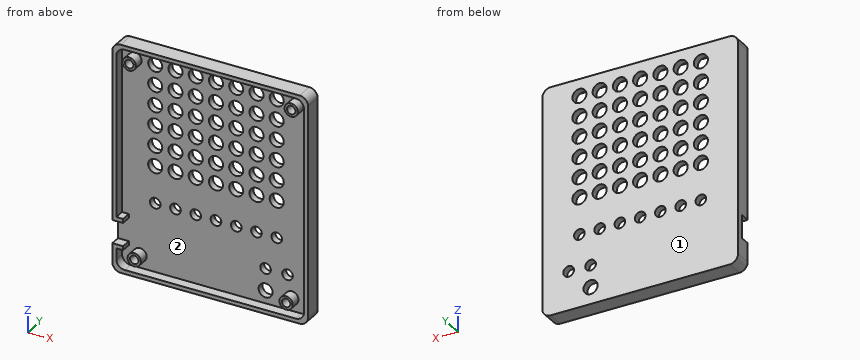
Autodesk Inventor part; units mm, degrees
ref_plane "YZ Plane" through (0, 0, 0) normal (1, 0, 0) x (0, 1, 0)
ref_plane "XZ Plane" through (0, 0, 0) normal (0, 1, 0) x (-1, 0, 0)
ref_plane "XY Plane" through (0, 0, 0) normal (0, 0, 1) x (1, 0, 0)
sketch "Sketch1" plane through (0, 0, 0) normal (0, 1, 0) x (-1, 0, 0)
  line L0 (-2.54, -83.185) -> (-71.12, -83.185) construction
  line L1 (-71.12, -83.185) -> (-71.12, -2.54) construction
  line L2 (-71.12, -2.54) -> (-2.54, -2.54) construction
  line L3 (-2.54, -2.54) -> (-2.54, -83.185) construction
  line L4 (0, -85.725) -> (-73.66, -85.725)
  line L5 (-73.66, -85.725) -> (-73.66, 0)
  line L6 (-73.66, 0) -> (0, 0)
  line L7 (0, 0) -> (0, -85.725)
  line L8 (-2.54, -83.185) -> (0, -85.725) construction
  line L9 (-71.12, -83.185) -> (-73.66, -85.725) construction
  line L10 (-73.66, 0) -> (-71.12, -2.54) construction
  line L11 (-2.54, -2.54) -> (0, 0) construction
  line L12 (-1.5, -84.225) -> (-72.16, -84.225)
  line L13 (-72.16, -84.225) -> (-72.16, -1.5)
  line L14 (-72.16, -1.5) -> (-1.5, -1.5)
  line L15 (-1.5, -1.5) -> (-1.5, -84.225)
  circle A0 centre (-8.255, -79.375) radius 1.6
  circle A1 centre (-65.405, -79.375) radius 1.6
  circle A2 centre (-6.35, -6.35) radius 1.6
  circle A3 centre (-67.31, -6.35) radius 1.6
  line L16 (-8.255, -79.375) -> (-65.405, -79.375) construction
  line L17 (-67.31, -6.35) -> (-6.35, -6.35) construction
  line L18 (-6.35, -6.35) -> (-8.255, -79.375) construction
  line L19 (-65.405, -79.375) -> (-67.31, -6.35) construction
  circle A4 centre (-8.255, -79.375) radius 2.5
  circle A5 centre (-65.405, -79.375) radius 2.5
  circle A6 centre (-67.31, -6.35) radius 2.5
  circle A7 centre (-6.35, -6.35) radius 2.5
  point P0 (0, 0)
  dimension "d0" = 68.58
  dimension "d1" = 80.645
  dimension "d2" = 2.54
  dimension "d3" = 2.54
  dimension "d4" = 1.5
  dimension "d5" = 57.15
  dimension "d6" = 60.96
  dimension "d7" = 73.025
  dimension "d9" = 3.81
  dimension "d10" = 3.81
  dimension "d11" = 3.81
  dimension "d12" = 3.2
  dimension "d13" = 5
extrude "Extrusion1" add sketch "Sketch1" along normal blind 2.54 contours L4 L5 L6 L7 | L12 L13 L14 L15 | A0 | A1 | A2 | A3 | A4 | A5 | A6 | A7
extrude "Extrusion2" add sketch "Sketch1" against normal blind 3.81
sketch "Sketch2" plane through (0, 0, 0) normal (0, -1, 0) x (1, 0, 0)
  circle A0 centre (67.31, -6.35) radius 2.5
  circle A1 centre (8.255, -79.375) radius 2.5
  line L0 (1.5, -1.5) -> (1.5, -84.225)
  line L1 (1.5, -84.225) -> (72.16, -84.225)
  line L2 (72.16, -84.225) -> (72.16, -1.5)
  line L3 (72.16, -1.5) -> (1.5, -1.5)
  circle A2 centre (65.405, -79.375) radius 2.5
  circle A3 centre (6.35, -6.35) radius 2.5
  circle A4 centre (59.69, -6.35) radius 2.65
  circle A5 centre (59.69, -13.97) radius 2.65
  circle A6 centre (59.69, -21.59) radius 2.65
  circle A7 centre (59.69, -29.21) radius 2.65
  circle A8 centre (59.69, -36.83) radius 2.65
  circle A9 centre (59.69, -44.45) radius 2.65
  circle A10 centre (52.07, -6.35) radius 2.65
  circle A11 centre (52.07, -13.97) radius 2.65
  circle A12 centre (52.07, -21.59) radius 2.65
  circle A13 centre (52.07, -29.21) radius 2.65
  circle A14 centre (52.07, -36.83) radius 2.65
  circle A15 centre (52.07, -44.45) radius 2.65
  circle A16 centre (44.45, -6.35) radius 2.65
  circle A17 centre (44.45, -13.97) radius 2.65
  circle A18 centre (44.45, -21.59) radius 2.65
  circle A19 centre (44.45, -29.21) radius 2.65
  circle A20 centre (44.45, -36.83) radius 2.65
  circle A21 centre (44.45, -44.45) radius 2.65
  circle A22 centre (36.83, -6.35) radius 2.65
  circle A23 centre (36.83, -13.97) radius 2.65
  circle A24 centre (36.83, -21.59) radius 2.65
  circle A25 centre (36.83, -29.21) radius 2.65
  circle A26 centre (36.83, -36.83) radius 2.65
  circle A27 centre (36.83, -44.45) radius 2.65
  circle A28 centre (29.21, -6.35) radius 2.65
  circle A29 centre (29.21, -13.97) radius 2.65
  circle A30 centre (29.21, -21.59) radius 2.65
  circle A31 centre (29.21, -29.21) radius 2.65
  circle A32 centre (29.21, -36.83) radius 2.65
  circle A33 centre (29.21, -44.45) radius 2.65
  circle A34 centre (21.59, -6.35) radius 2.65
  circle A35 centre (21.59, -13.97) radius 2.65
  circle A36 centre (21.59, -21.59) radius 2.65
  circle A37 centre (21.59, -29.21) radius 2.65
  circle A38 centre (21.59, -36.83) radius 2.65
  circle A39 centre (21.59, -44.45) radius 2.65
  circle A40 centre (13.97, -6.35) radius 2.65
  circle A41 centre (13.97, -13.97) radius 2.65
  circle A42 centre (13.97, -21.59) radius 2.65
  circle A43 centre (13.97, -29.21) radius 2.65
  circle A44 centre (13.97, -36.83) radius 2.65
  circle A45 centre (13.97, -44.45) radius 2.65
  circle A46 centre (59.69, -58.3946) radius 2
  circle A47 centre (52.07, -58.3946) radius 2
  circle A48 centre (44.45, -58.3946) radius 2
  circle A49 centre (36.83, -58.3946) radius 2
  circle A50 centre (29.21, -58.3946) radius 2
  circle A51 centre (21.59, -58.3946) radius 2
  circle A52 centre (13.97, -58.3946) radius 2
  line L4 (67.31, -6.35) -> (59.69, -6.35) construction
  line L5 (65.405, -79.375) -> (59.69, -58.3946) construction
  line L6 (13.97, -58.3946) -> (8.255, -79.375) construction
  circle A53 centre (55.499, -79.375) radius 2.65
  line L7 (55.499, -79.375) -> (65.405, -79.375) construction
  circle A54 centre (55.499, -71.1454) radius 2
  circle A55 centre (63.754, -71.1454) radius 2
  line L8 (55.499, -71.1454) -> (63.754, -71.1454) construction
  line L9 (55.499, -71.1454) -> (55.499, -79.375) construction
  point P0 (0, 0)
  dimension "d20" = 7.62
  dimension "d23" = 7.62
  dimension "d26" = 5.3
  dimension "d29" = 7.62
  dimension "d34" = 7.62
  dimension "d35" = 7.62
  dimension "d36" = 60.96
  dimension "d37" = 20.9804
  dimension "d38" = 4
  dimension "d40" = 9.906
  dimension "d41" = 8.255
  dimension "d42" = 8.2296
extrude "Extrusion3" cut sketch "Sketch2" against normal through all contours A4 | A5 | A6 | A7 | A8 | A9 | A10 | A11 | A12 | A13 | A14 | A15 | A16 | A17 | A18 | A19 | A20 | A21 | A22 | A23 | A24 | A25 | A26 | A27 | A28 | A29 | A30 | A31 | A32 | A33 | A34 | A35 | A36 | A37 | A38 | A39 | A40 | A41 | A42 | A43 | A44 | A45 | A46 | A47 | A48 | A49 | A50 | A51 | A52 | A53 | A54 | A55
sketch "Sketch3" plane through (0, 0, 0) normal (0, -1, 0) x (1, 0, 0)
  line L0 (1.5, -1.5) -> (1.5, -84.225)
  line L1 (1.5, -75.4634) -> (0, -75.4634)
  line L2 (0, -75.4634) -> (0, -66.7512)
  line L3 (0, -66.7512) -> (1.5, -66.7512)
  line L4 (1.5, -66.7512) -> (1.5, -75.4634)
  line L5 (0, -85.725) -> (73.66, -85.725)
  line L6 (2.54, -83.185) -> (71.12, -83.185) construction
  line L7 (2.54, -2.54) -> (2.54, -83.185) construction
  line L8 (1.5, -75.4634) -> (4.04, -75.4634)
  line L9 (4.04, -75.4634) -> (4.04, -76.9874)
  line L10 (4.04, -76.9874) -> (1.5, -76.9874)
  line L11 (1.5, -76.9874) -> (1.5, -75.4634)
  line L12 (1.5, -66.7512) -> (4.04, -66.7512)
  line L13 (4.04, -66.7512) -> (4.04, -65.2272)
  line L14 (4.04, -65.2272) -> (1.5, -65.2272)
  line L15 (1.5, -65.2272) -> (1.5, -66.7512)
  line L16 (4.04, -66.7512) -> (4.04, -75.4634) construction
  point P0 (0, 0)
  dimension "d46" = 8.7122
  dimension "d49" = 7.7216
  dimension "d50" = 1.524
  dimension "d53" = 2.54
extrude "Extrusion4" cut sketch "Sketch3" along normal through all contours L0 L1 L2 L3
extrude "Extrusion5" add sketch "Sketch3" along normal up to surface (3.81 mm away) contours L14 L13 L12 L0 | L8 L9 L10 L0
fillet "Fillet1" radius 3.175 8 edges at (1.5, -1.905, -84.225) (0, -0.635, -85.725) (73.66, -0.635, -85.725) (72.16, -1.905, -84.225) (72.16, -1.905, -1.5) (73.66, -0.635, 0) (1.5, -1.905, -1.5) (0, -0.635, 0)
properties part number "Top Part"
Can you work these out from the model? Positions are in its coordinate system, mm. Face numbers are marked on the shaded views. Round coordinates to 2 decimals unless told otherwise and drop trailing zeros. Loops run counter-clockwise (first coordinate to the right, second up) from the corner with the lowest first, then second, coordinate; pieces in that order, holes last. Notation, with made-up numbers: M -13,8.5 L 17,8.5 A19 ccw 17,19.5 Z; hole C 79.5,8.25 d3. An arc over 180 degrees is marked long. Answer as a JSON object with one key per item and string values. Group by question number.
Q1. Please list where these lines run through material, in increasing order: L1, parallel to X at y = -2.75, z = -18.5; L2, parallel to Z at x = 21, y = -1.25 (3 decimals); L3, parallel to X at y = -3, z = -5.5.
Q2. Imagine slicing it at B-B, the plane z = -51. Please give me the cut outline in (x, y), then the cut area to 3 significant figures.
Q3. Will this pin go through, and if not, where does the flat tip stop? pin 1 (12 mm diameter, centred on x = 62.5, z = -30.5, fed in from -Y).
Q4. Imagine slicing it at A-A, the plane y = -1.5. Count the separate pieces of the cut face and the enclosed holes in it, then the cut area to 3 significant figures.
Q5. We'd pull the mould along Z, two halves only. Please class the marked faces 1 and 2: +Z half, -Z half, draft (parallel to the pull), parting line (faces both ways), or undercut.
Findings:
{
 "1": {"L1": "x = 0 to 1.5, 72.16 to 73.66", "L2": "z = -85.725 to -84.225, -1.5 to 0", "L3": "x = 0 to 1.5, 4 to 4.99, 7.71 to 8.7, 64.96 to 65.95, 68.67 to 69.66, 72.16 to 73.66"},
 "2": {"outline": "M 0,-3.81 L 1.5,-3.81 L 1.5,0 L 72.16,0 L 72.16,-3.81 L 73.66,-3.81 L 73.66,2.54 L 0,2.54 Z", "area": "199 mm2"},
 "3": {"pin 1": "stops at y = 0"},
 "4": {"separate pieces": "5", "enclosed holes": "4", "area": "510 mm2"},
 "5": {"face 1": "draft", "face 2": "undercut"}
}
